Autodesk Inventor part; units mm, degrees
ref_plane "YZ Plane" through (0, 0, 0) normal (1, 0, 0) x (0, 1, 0)
ref_plane "XZ Plane" through (0, 0, 0) normal (0, 1, 0) x (-1, 0, 0)
ref_plane "XY Plane" through (0, 0, 0) normal (0, 0, 1) x (1, 0, 0)
sketch "Szkic1" plane through (0, 0, 0) normal (0, 0, 1) x (1, 0, 0)
  circle A0 centre (0, 0) radius 25
  circle A1 centre (0, 0) radius 7
  line L0 (-24, 30) -> (24, 30)
  line L1 (30, 24) -> (30, -24)
  line L2 (24, -30) -> (-24, -30)
  line L3 (-30, -24) -> (-30, 24)
  line L4 (-30, 30) -> (30, -30) construction
  line L5 (30, 30) -> (-30, -30) construction
  circle A2 centre (-24.7487, 24.7487) radius 2.75
  circle A3 centre (24.7487, 24.7487) radius 2.75
  circle A4 centre (-24.7487, -24.7487) radius 2.75
  circle A5 centre (24.7487, -24.7487) radius 2.75
  arc A6 (-24, 30) -> (-30, 24) centre (-24, 24) ccw
  arc A7 (30, 24) -> (24, 30) centre (24, 24) ccw
  arc A8 (24, -30) -> (30, -24) centre (24, -24) ccw
  arc A9 (-30, -24) -> (-24, -30) centre (-24, -24) ccw
  dimension "d0" = 50
  dimension "d1" = 14
  dimension "d2" = 60
  dimension "d3" = 60
  dimension "d5" = 5.5
  dimension "d6" = 5.5
  dimension "d7" = 5.5
  dimension "d8" = 5.5
  dimension "d9" = 6
extrude "Wyciągnięcie proste1" add sketch "Szkic1" along normal blind 7 contours A0 | A1 | L0 A7 L1 A8 L2 A9 L3 A6
extrude "Wyciągnięcie proste2" add sketch "Szkic1" against normal blind 3 contours A0
extrude "Wyciągnięcie proste3" add sketch "Szkic1" against normal blind 30 contours A1
sketch "Szkic2" plane through (0, 0, 7) normal (0, 0, 1) x (1, 0, 0)
  line L0 (-30, 12.4264) -> (-12.4264, 30)
  line L1 (12.4264, 30) -> (30, 12.4264)
  line L2 (30, -12.4264) -> (12.4264, -30)
  line L3 (-12.4264, -30) -> (-30, -12.4264)
  line L4 (-30, 30) -> (30, -30) construction
  line L5 (30, 30) -> (-30, -30) construction
  line L6 (-12.4264, 30) -> (12.4264, 30)
  line L7 (30, -24) -> (30, 24)
  line L8 (30, 12.4264) -> (30, -12.4264)
  line L9 (-24, -30) -> (24, -30)
  line L10 (12.4264, -30) -> (-12.4264, -30)
  line L11 (-30, 24) -> (-30, -24)
  line L12 (-30, -12.4264) -> (-30, 12.4264)
  point P0 (0, 0)
extrude "Wyciągnięcie proste4" add sketch "Szkic2" along normal blind 65.5
fillet "Zaokrąglenie1" radius 2 8 edges at (30, 0, 72.5) (21.2132, 21.2132, 72.5) (0, 30, 72.5) (-21.2132, 21.2132, 72.5) (-30, 0, 72.5) (21.2132, -21.2132, 72.5) (0, -30, 72.5) (-21.2132, -21.2132, 72.5)
chamfer "Faza1" distance 1 angle 45 1 edges at (-7, 0, -30)
properties part number "silnik_podstawa" material "Aluminium 6061-AHC"
Verification items for the finished model (mm, model axes). A direction names the side the tool comes from. Coordinates: 2 decimals unless noted, no trailing zeros. Loops run counter-clockwise (first coordinate to the right, second up) from the corner with the lowest first, then second, coordinate; pieces in that order, holes last. Notation, with made-up numbers: (21.25, 87.25) -> (79.25, 87.25) arc R23 ccw to (79.25, 108.25) -> close; hole circle Ø10 at (-22.5, 73). An arc over 180 degrees is marked (long way). Answer in a Markdown table with one row per item. Add a question column.
1. Depth check by flat-ended pin: P1, Ø6.5, axis at x = 24.75, y = 24.75, coming from the -Z side; P2, Ø14, axis at x = 22, y = 23, coming from the +Z side; P3, Ø6.5, axis at x = -24.75, y = 24.75, coming from the +Z side; P4, Ø18, axis at x = 13.5, y = 9, coming from the -Z side. Enter the tip coordinate at first touch or a pass-through.
2. Section check A-A, the plane x = 0. Enter the section's corners in (y, z).
3. Section check B-B, the plane z = 65. Enter the section's corners in (x, y), then the cut area to 3 significant figures.
4. Section check D-D, the plane y = 10. Enter the section's corners in (x, z).
5. Access from +Z, -Z, +X, -X, +Y, -Y to the whole of each face (thin tool, end or side, straight path). Record for faces 1 (the face through (6.466, -2.681, -15.818)), 2 (the face through (23.8, 21.9, 7)), 3 (the face through (21.336, -21.09, 38.306)).
6. Draft check along Y on faces 4 (the face through (0, 0, -30)), 5 (the face through (-28.196, -28.289, 3.451)), 6 (the face through (24.153, 27.433, 3.451)). Enter one of: +Y half, -Y half, draft (parallel to the pull), parting line (faces both ways), or undercut.
7. Material ranges on probe 1 along Z at (x, y) = (7.5, 13); probe 2 along Z at (x, y) = (-26.5, 10.5); probe 3 along X at (y, z) = (13, 59), recorded low to high. Write a range as [from, to].
Derived:
| question | item | result |
|---|---|---|
| 1 | P1 | stops at z = 0 |
| 1 | P2 | stops at z = 72.5 |
| 1 | P3 | stops at z = 7 |
| 1 | P4 | stops at z = -3 |
| 2 | outline | (-30, 0) -> (-25, 0) -> (-25, -3) -> (-7, -3) -> (-7, -29) -> (-6, -30) -> (6, -30) -> (7, -29) -> (7, -3) -> (25, -3) -> (25, 0) -> (30, 0) -> (30, 70.5) arc R2 ccw to (28, 72.5) -> (-28, 72.5) arc R2 ccw to (-30, 70.5) -> close |
| 3 | outline | (-30, -12.43) -> (-12.43, -30) -> (12.43, -30) -> (30, -12.43) -> (30, 12.43) -> (12.43, 30) -> (-12.43, 30) -> (-30, 12.43) -> close |
| 3 | area | 2,980 mm² |
| 4 | outline | (-30, 0) -> (-22.91, 0) -> (-22.91, -3) -> (22.91, -3) -> (22.91, 0) -> (30, 0) -> (30, 70.5) arc R2 ccw to (28, 72.5) -> (-28, 72.5) arc R2 ccw to (-30, 70.5) -> close |
| 5 | face 1 | -Z |
| 5 | face 2 | +Z, +X, +Y |
| 5 | face 3 | +Z, +X, -Y |
| 6 | face 4 | draft |
| 6 | face 5 | -Y half |
| 6 | face 6 | undercut |
| 7 | probe 1 | z = [-3, 72.5] |
| 7 | probe 2 | z = [0, 72.5] |
| 7 | probe 3 | x = [-29.43, 29.43] |
